```python
from build123d import *

# Parameters (mm, degrees)
F1_DEPTH = 3
F2_R     = 1
F3_R     = 1.25
F4_DEPTH = 1
F6_DEPTH = 1.5


with BuildPart() as f1:
    # F0 (on Top) → F1 (new body)
    with BuildSketch(Plane.XY):
        Polygon((0, 55.125), (-34.43, 0), (34.43, 0), align=None)
        Polygon((-5.15597, 34.647), (5.15597, 34.647), (17.74764, 14.486798), (17.06, 10.587), (-17.06, 10.587), (-17.74764, 14.486798), align=None, mode=Mode.SUBTRACT)
    extrude(amount=F1_DEPTH)

    # F2
    f2_edges = [f1.edges().sort_by_distance(p)[0] for p in [
        (17.06, 10.587, 1.5),
        (-17.06, 10.587, 1.5),
        (17.74764, 14.486798, 1.5),
        (-17.74764, 14.486798, 1.5),
        (5.15597, 34.647, 1.5),
        (-5.15597, 34.647, 1.5),
    ]]
    fillet(f2_edges, radius=F2_R)

    # F3 (on face) → F4 (cut)
    with BuildSketch(Plane.XY.offset(3)):
        with Locations((0, 47.652587)):
            Circle(F3_R)
    extrude(amount=-F4_DEPTH, mode=Mode.SUBTRACT)

    # F5 (on face) → F6 (join)
    with BuildSketch(Plane(origin=(0, 0, 0), x_dir=(1, 0, 0), z_dir=(0, 0, -1))):
        Polygon((20.099395, -15.818272), (20.426854, -14.132703), (19.694041, -9.976712), (17.20362, -7.887), (-17.20362, -7.887), (-19.694041, -9.976712), (-20.426854, -14.132703), (-20.099395, -15.818272), (-7.369729, -36.199417), (-5.299942, -37.347), (5.299942, -37.347), (7.369729, -36.199417), align=None)
        Polygon((4.342852, -33.647), (-4.342852, -33.647), (-4.738556, -33.427604), (-16.598042, -14.439682), (-16.664021, -14.10006), (-16.284103, -11.945441), (-15.85693, -11.587), (15.85693, -11.587), (16.284103, -11.945441), (16.664021, -14.10006), (16.598042, -14.439682), (4.738556, -33.427604), align=None, mode=Mode.SUBTRACT)
    extrude(amount=-F6_DEPTH)


solid = f1.part
```
Build history of the part. All positions in model axes, mm. A direction names the side the tool comes from. Give positions to 0.01 mm unless a question says otherwise; leave off trailing zeros. Order: outer loops, then holes, each group sorted by start corner. A loop starts at its lowest first (then second) coordinate and runs counter-clockwise, first axis right, second up. Notation, with made-up numbers: M 32.5,40.5 L 87.5,40.5 A21 cw 87.5,78.5 Z; hole C -15.5,22 d8. An arc over 180 degrees is marked long. Return JSON: item names as keys, results as strings.
Q1. Flat gauge pins, fed straight in: pin 1 (1 mm diameter, centred on y = 17, z = 2, fed in from -X); pin 2 (1.5 mm diameter, centred on y = 42.5, z = 2.5, fed in from -X); pin 3 (1.2 mm diameter, centred on x = -1.5, z = 2, fed in from +Y). Where does each tip first touch, or does it go through?
Answer list:
{"pin 1": "stops at x = -24.12", "pin 2": "stops at x = -8.35", "pin 3": "stops at y = 53.68"}
Q2. Band-saw the part on C-C (x = -11.5). Give the cut face in (y, z).
Answer list:
{"outline": "M 0,0 L 11.59,0 L 11.59,1.5 L 10.59,1.5 L 10.59,3 L 0,3 Z; M 22.6,0 L 36.71,0 L 36.71,3 L 24.49,3 L 24.49,1.5 L 22.6,1.5 Z"}
Q3. Two-plate mould, pull along Y, no slides. Class faces 1 (the face through (-17.44, 12.74, 2.24)), 2 (the face through (-16.974, 27.948, 1.479)), 3 (the face through (0, 10, 0)): pulls with the +Y half, pulls with the -Y half, needs draft (parallel to the pull), parting line crosses it, or undercut.
Answer list:
{"face 1": "undercut", "face 2": "pulls with the +Y half", "face 3": "needs draft"}
Q4. Band-saw the part on A-A (z = 0.65). Give the cut face in (x, y) (3 decimals), then the cut area to 3 significant figures.
Answer list:
{"outline": "M -34.43,0 L 34.43,0 L 0,55.125 Z; hole M -16.664,14.1 L -16.284,11.945 L -15.857,11.587 L 15.857,11.587 L 16.284,11.945 L 16.664,14.1 L 16.598,14.44 L 4.739,33.428 L 4.343,33.647 L -4.343,33.647 L -4.739,33.428 L -16.598,14.44 Z", "area": "1,400 mm^2"}
Q5. Band-saw the part on B-B (y = 32.5). Give the cut face in (x, z), then the cut area to 3 significant figures.
Answer list:
{"outline": "M -14.13,0 L -5.32,0 L -5.32,1.5 L -6.5,1.5 L -6.5,3 L -14.13,3 Z; M 5.32,0 L 14.13,0 L 14.13,3 L 6.5,3 L 6.5,1.5 L 5.32,1.5 Z", "area": "49.3 mm^2"}
Q6. Band-saw the part on D-D (x = 26). Give the cut face in (y, z).
Answer list:
{"outline": "M 0,0 L 13.5,0 L 13.5,3 L 0,3 Z"}
Q7. Wall check: probe 1 along Y at (x, z) = (7, 2.2); probe 2 along X at (y, z) = (21, 1.4); probe 3 along X at (y, z) = (22.5, 1.2). Give the ranges that are in metal, low to high. Write a range as from..to.
Answer list:
{"probe 1": "y = 0..10.59, 31.69..43.92", "probe 2": "x = -21.31..-12.5, 12.5..21.31", "probe 3": "x = -20.38..-11.56, 11.56..20.38"}
Q8. 3-axis set-ups, long thin cutter, end or side, ignore diameter. For faces 4 (the face through (0, 11.587, 1)), 5 (the face through (-11.58, 24.36, 2.24)), 6 (the face through (17.456, 27.177, 1.479)): which of +Z, -Z, +X, -X, +Y, -Y reach the whole face in a straight line?
Answer list:
{"face 4": "+Z, -Z", "face 5": "+Z", "face 6": "+Z, -Z, +X, +Y"}
